For this review, take the finished solid that the model builds, in its own axes (mm). Coordinates: 2 decimals unless noted, no trailing zeros. Loops run counter-clockwise (first coordinate to the right, second up) from the corner with the lowest first, then second, coordinate; pieces in that order, holes last. Notation, with made-up numbers: M 74.25,47 L 113.25,47 A23 ccw 113.25,84 Z; hole C 23.5,-28 d7. An arc over 180 degrees is marked long. Put each result on its own line as item: value.
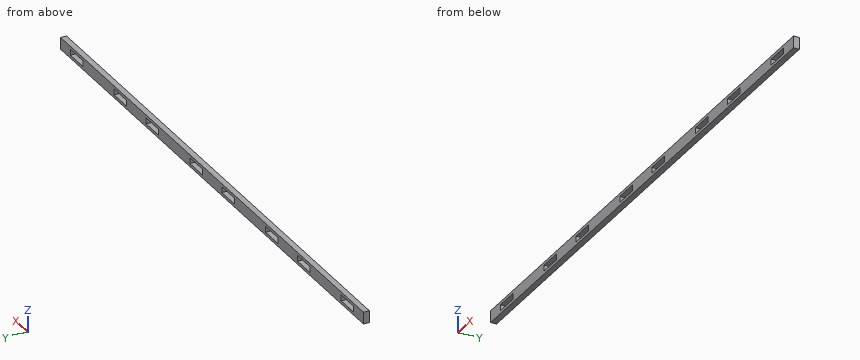
```python
from build123d import *

# Parameters (mm, degrees)
SKETCH1_W           = 615.917267528
SKETCH1_H           = 12.7
BOSS_EXTRUDE1_DEPTH = 6.35
SKETCH2_W           = 25.4
SKETCH2_H           = 6.35
CUT_EXTRUDE1_DEPTH  = 7.35
LPATTERN1_COUNT     = 2
LPATTERN1_PITCH     = 307.958633764
LPATTERN1_COL_COUNT = 2
LPATTERN1_COL_PITCH = 307.958633764


with BuildPart() as part:
    # Sketch1 → Boss-Extrude1 (new body)
    with BuildSketch(Plane(origin=(0, 0, 0), x_dir=(1, 0, 0), z_dir=(0, 1, 0))):
        Rectangle(SKETCH1_W, SKETCH1_H)
    extrude(amount=BOSS_EXTRUDE1_DEPTH)

    # Sketch2 → Cut-Extrude1 (cut, through all)
    with BuildSketch(Plane(origin=(0, 6.35, 0), x_dir=(1, 0, 0), z_dir=(0, 1, 0))):
        with Locations((-32.539658441, 0)):
            Rectangle(SKETCH2_W, SKETCH2_H)
        with Locations((32.539658441, 0)):
            Rectangle(SKETCH2_W, SKETCH2_H)
        with Locations((-121.439658441, 0)):
            Rectangle(SKETCH2_W, SKETCH2_H)
        with Locations((121.439658441, 0)):
            Rectangle(SKETCH2_W, SKETCH2_H)
    cut_extrude1 = extrude(amount=-CUT_EXTRUDE1_DEPTH, mode=Mode.SUBTRACT)

    # LPattern1: Cut-Extrude1 ×2
    with Locations(*[(i * LPATTERN1_PITCH, 0, 0) for i in range(1, LPATTERN1_COUNT)]):
        add(cut_extrude1, mode=Mode.SUBTRACT)

    # LPattern1 col: Cut-Extrude1 ×2
    with Locations(*[(-i * LPATTERN1_COL_PITCH, 0, 0) for i in range(1, LPATTERN1_COL_COUNT)]):
        add(cut_extrude1, mode=Mode.SUBTRACT)


solid = part.part
```
(1) Add section A-A (x = 119). Write out the cut boundary in (y, z) (3 decimals).
Determined:
outline: M 0,-6.35 L 6.35,-6.35 L 6.35,-3.175 L 0,-3.175 Z; M 0,3.175 L 6.35,3.175 L 6.35,6.35 L 0,6.35 Z
(2) Add section B-B (y = 1.75). State how many separate pieces and enclosed holes the cut face has, plus the area to 3 significant figures.
Determined:
separate pieces: 1
enclosed holes: 8
area: 6,530 mm^2
(3) Wall thickness on line 1 along Z through (x, y) = (23, 4.5) (3 decimals): over which ranges is the line inside the solid? List them lowest first. Write a range as [from, to].
Determined:
line 1: z = [-6.35, -3.175], [3.175, 6.35]
